Autodesk Inventor part; units mm, degrees
ref_plane "YZ Plane" through (0, 0, 0) normal (1, 0, 0) x (0, 1, 0)
ref_plane "XZ Plane" through (0, 0, 0) normal (0, 1, 0) x (-1, 0, 0)
ref_plane "XY Plane" through (0, 0, 0) normal (0, 0, 1) x (1, 0, 0)
sketch "Sketch1" plane through (0, 0, 0) normal (0, 1, 0) x (-1, 0, 0)
  line L0 (-8.55, 8.55) -> (8.55, 8.55)
  line L1 (8.55, 8.55) -> (8.55, -8.55)
  line L2 (8.55, -8.55) -> (-8.55, -8.55)
  line L3 (-8.55, -8.55) -> (-8.55, 8.55)
  line L4 (-8.55, 8.55) -> (8.55, -8.55) construction
  line L5 (8.55, 8.55) -> (-8.55, -8.55) construction
  line L6 (7.55, 7.55) -> (-7.55, 7.55)
  line L7 (-7.55, 7.55) -> (-7.55, -7.55)
  line L8 (-7.55, -7.55) -> (7.55, -7.55)
  line L9 (7.55, -7.55) -> (7.55, 7.55)
  line L10 (7.55, 7.55) -> (-7.55, -7.55) construction
  line L11 (-7.55, 7.55) -> (7.55, -7.55) construction
  line L12 (1.5, 2.35) -> (-1.5, 2.35)
  line L13 (-1.5, 2.35) -> (-1.5, 3.35)
  line L14 (-1.5, 3.35) -> (1.5, 3.35)
  line L15 (1.5, 3.35) -> (1.5, 2.35)
  line L16 (1.5, 2.35) -> (-1.5, 3.35) construction
  line L17 (-1.5, 2.35) -> (1.5, 3.35) construction
  line L18 (1.5, -3.35) -> (-1.5, -3.35)
  line L19 (-1.5, -3.35) -> (-1.5, -2.35)
  line L20 (-1.5, -2.35) -> (1.5, -2.35)
  line L21 (1.5, -2.35) -> (1.5, -3.35)
  line L22 (1.5, -3.35) -> (-1.5, -2.35) construction
  line L23 (-1.5, -3.35) -> (1.5, -2.35) construction
  line L24 (0, 0) -> (-1, 0)
  circle A0 centre (-6.3, 6.3) radius 1.25
  circle A1 centre (-6.3, 6.3) radius 2.25
  circle A2 centre (-6.3, -6.3) radius 1.25
  circle A3 centre (-6.3, -6.3) radius 2.25
  circle A4 centre (6.3, -6.3) radius 1.25
  circle A5 centre (6.3, -6.3) radius 2.25
  circle A6 centre (6.3, 6.3) radius 1.25
  circle A7 centre (6.3, 6.3) radius 2.25
  point P0 (0, 2.85)
  point P1 (0, -2.85)
  point P2 (-8.55, 6.3)
  point P3 (-8.55, -6.3)
  point P4 (-6.3, -8.55)
  point P5 (6.3, -8.55)
  point P6 (8.55, -6.3)
  point P7 (8.55, 6.3)
  point P8 (6.3, 8.55)
  point P9 (-6.3, 8.55)
  point P10 (-7.55, 6.3)
  point P11 (-6.3, 7.55)
  point P12 (6.3, 7.55)
  point P13 (7.55, 6.3)
  point P14 (7.55, -6.3)
  point P15 (6.3, -7.55)
  point P16 (-6.3, -7.55)
  point P17 (-7.55, -6.3)
  dimension "d0" = 17.1
  dimension "d1" = 17.1
  dimension "d4" = 1
  dimension "d5" = 1
  dimension "d6" = 5.7
  dimension "d7" = 3
  dimension "d8" = 1
  dimension "d10" = 2.5
extrude "Extrusion2" add sketch "Sketch1" along normal blind 1 contours L0 A7 L6 A1 | A1 L6 L7 | A1 L7 A3 L3 | A7 L9 L6 | A1 L7 A0 L6 | L6 A7 L9 A5 L8 A3 L7 A1 | A3 L7 L8 | L1 A5 L9 A7 | L6 A6 L9 A7 | A0 L7 L6 | A0 | A3 L8 A2 L7 | A3 L8 A5 L2 | A5 L8 L9 | L6 L9 A6 | A6 | A2 L8 L7 | A2 | L9 A4 L8 A5 | A4 | L9 L8 A4 | L12 L13 L14 L15 | L18 L19 L20 L21
extrude "Extrusion3" add sketch "Sketch1" against normal blind 2 contours L0 A7 L6 A1 | A1 L6 L7 | A1 L7 A3 L3 | A7 L9 L6 | A3 L7 L8 | L1 A5 L9 A7 | A0 L7 L6 | A3 L8 A5 L2 | A5 L8 L9 | L6 L9 A6 | A2 L8 L7 | L9 L8 A4
extrude "Extrusion4" add sketch "Sketch1" against normal blind 3 contours L12 L13 L14 L15 | L18 L19 L20 L21
properties part number "keycap"
Geometry check sheet. Reference: the model listing, model coordinates, mm. A direction names the side the tool comes from. Round coordinates to 2 decimals unless told otherwise and drop trailing zeros. Loops run counter-clockwise (first coordinate to the right, second up) from the corner with the lowest first, then second, coordinate; pieces in that order, holes last. Notation, with made-up numbers: (-2, 26.5) -> (10, 26.5) arc R23 cw to (10, 54.5) -> close; hole circle Ø11 at (25, -24.75). An arc over 180 degrees is marked (long way). Answer as a JSON object with one key per item and string values. Group by question number.
Item 1: Release check for a two-part mould opening along Z. For faces 3 (the face through (0, 0, 0)), 4 (the face through (8.55, -1, 0)), 5 (the face through (0, -1, -8.55)) record: pulls with the +Z half, pulls with the -Z half, needs draft (parallel to the pull), parting line crosses it, or undercut.
Item 2: Cross-section at B-B, the plane x = 0.25. Record the cut outline in (y, z), plus the area to 3 significant figures.
Item 3: Set-up check for faces 1 (the face through (1.5, -1, 3)), 2 (the face through (7.91, -0.52, 7.87)): record each of +Z, -Z, +X, -X, +Y, -Y from which the full face is reachable in a straight line by a thin tool's end or side.
Item 4: Depth check by flat-ended pin: pin 1 Ø8.5 at (x, z) = (2.5, 3) entering from -Y. Enter the tip coordinate at first touch or a pass-through.
Item 5: Cross-section at A-A, the plane y = -0.3. Record the cut outline in (x, z), plus the area to 3 significant figures.
Item 6: Thickness scan on line 1 along Z through (x, y) = (-1.25, -0.05); line 2 along Z through (x, y) = (1.75, -1.05). Record the ranges inside material, lowest first.
Item 7: Cross-section at C-C, the plane z = -5.25. Record the cut outline in (x, y), plus the area to 3 significant figures.
Item 8: Cross-section at D-D, the plane x = 3.75. Record the cut outline in (y, z).
Determined:
{
 "1": {"face 3": "undercut", "face 4": "needs draft", "face 5": "pulls with the -Z half"},
 "2": {"outline": "(-3, -3.35) -> (0, -3.35) -> (0, -7.55) -> (-2, -7.55) -> (-2, -8.55) -> (1, -8.55) -> (1, 8.55) -> (-2, 8.55) -> (-2, 7.55) -> (0, 7.55) -> (0, 3.35) -> (-3, 3.35) -> (-3, 2.35) -> (0, 2.35) -> (0, -2.35) -> (-3, -2.35) -> close", "area": "27.1 mm²"},
 "3": {"face 1": "-Y", "face 2": "+Z, +X, +Y, -Y"},
 "4": {"pin 1": "stops at y = -3"},
 "5": {"outline": "(-8.55, -6.3) arc R2.25 ccw to (-6.3, -8.55) -> (6.3, -8.55) arc R2.25 ccw to (8.55, -6.3) -> (8.55, 6.3) arc R2.25 ccw to (6.3, 8.55) -> (-6.3, 8.55) arc R2.25 ccw to (-8.55, 6.3) -> close; (-1.5, -3.35) -> (1.5, -3.35) -> (1.5, -2.35) -> (-1.5, -2.35) -> close; (-1.5, 2.35) -> (1.5, 2.35) -> (1.5, 3.35) -> (-1.5, 3.35) -> close; hole (-7.55, -6.3) arc R1.25 ccw to (-6.3, -7.55) -> (6.3, -7.55) arc R1.25 ccw to (7.55, -6.3) -> (7.55, 6.3) arc R1.25 ccw to (6.3, 7.55) -> (-6.3, 7.55) arc R1.25 ccw to (-7.55, 6.3) -> close", "area": "67.4 mm²"},
 "6": {"line 1": "z = -8.55 to -7.55, -3.35 to -2.35, 2.35 to 3.35, 7.55 to 8.55", "line 2": "z = -8.55 to -7.55, 7.55 to 8.55"},
 "7": {"outline": "(-8.55, -2) -> (-7.55, -2) -> (-7.55, 0) -> (7.55, 0) -> (7.55, -2) -> (8.55, -2) -> (8.55, 1) -> (-8.55, 1) -> close", "area": "21.1 mm²"},
 "8": {"outline": "(-2, -8.55) -> (1, -8.55) -> (1, 8.55) -> (-2, 8.55) -> (-2, 7.55) -> (0, 7.55) -> (0, -7.55) -> (-2, -7.55) -> close"}
}
